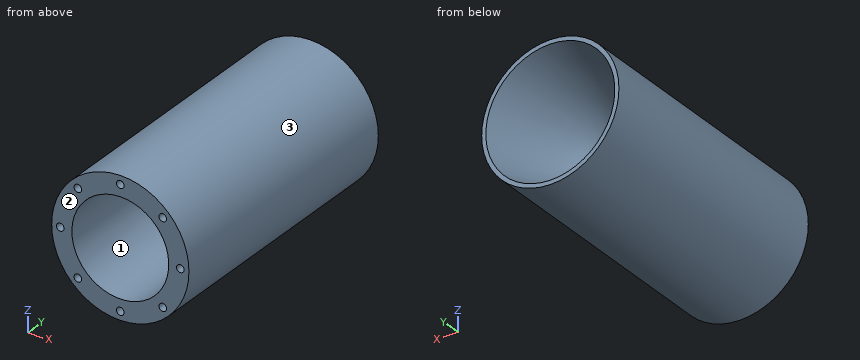
from build123d import *

# Parameters (mm, degrees)
SHORTEN_CHAMBER_75IN_BY = 19.05
CIRPATTERN1_COUNT       = 8


with BuildPart() as part:
    # Sketch1 → Revolve2 (revolve)
    with BuildSketch(Plane.XY, mode=Mode.PRIVATE) as revolve2_sk:
        with BuildLine():
            Line((71.638455479, 109.927347077), (76.2, 109.927347077))
            Line((76.2, 109.927347077), (76.2, -212.127673725))
            Line((76.2, -212.127673725), (53.792460196, -212.127673725))
            Line((53.792460196, -212.127673725), (53.792460196, -59.727673725))
            add(Edge.make_bspline(
                [(53.792460196, -59.727673725), (53.792458964, -59.657143655), (53.791929819, -59.515566601), (53.789553965, -59.181725115), (53.783229362, -58.904955991), (53.77374387, -58.532727986), (53.761100968, -58.21299812), (53.741350135, -57.781754942), (53.711337787, -57.281120398), (53.667125616, -56.688158665), (53.588220936, -55.848640867), (53.488359334, -55.008326363), (53.367608248, -54.172595934), (53.197743271, -53.172585746), (53.002996623, -52.17760333), (52.777307543, -51.188699595), (52.520946634, -50.207649553), (52.240221737, -49.233238259), (51.935281123, -48.266129746), (51.5444702, -47.149295595), (51.050452714, -45.89056894), (50.509666089, -44.651129345), (49.922993248, -43.432862075), (49.291052535, -42.237253796), (48.615057518, -41.066315445), (47.895407794, -39.921133233), (47.134034398, -38.804236825), (46.430801308, -37.85161238), (45.804470174, -37.055832726), (45.263749909, -36.403541893), (44.82605917, -35.894408249), (44.425708405, -35.447153279), (44.092389714, -35.084791811), (43.784856831, -34.760500781), (43.58500461, -34.551710083), (43.355324273, -34.318676923), (43.254715351, -34.217322692), (43.204843203, -34.167450306)],
                knots=[0.082637729, 0.082637729, 0.082637729, 0.082637729, 0.082637729, 0.092574926, 0.102512123, 0.11244932, 0.122386517, 0.132323714, 0.142260911, 0.162135305, 0.182009699, 0.201884093, 0.24163288, 0.261507274, 0.281381668, 0.321130456, 0.360879243, 0.380753637, 0.400628031, 0.440376819, 0.480125606, 0.519874394, 0.559623181, 0.599371969, 0.639120757, 0.678869544, 0.718618332, 0.75836712, 0.798115907, 0.817990301, 0.837864695, 0.857739089, 0.877613483, 0.88755068, 0.897487877, 0.907425074, 0.91736227, 0.91736227, 0.91736227, 0.91736227, 0.91736227], degree=4))
            Line((43.204843203, -34.167450306), (34.597215006, -25.55982211))
            add(Edge.make_bspline(
                [(24.01, 0), (24.010001231, -0.070528647), (24.010530378, -0.21358419), (24.012906064, -0.543182916), (24.019230459, -0.824160397), (24.028715581, -1.194822072), (24.041357875, -1.513435058), (24.0571581, -1.861939603), (24.076113359, -2.193706872), (24.103750974, -2.6180694), (24.143219182, -3.122033947), (24.214231845, -3.879978675), (24.334058818, -4.886450388), (24.510418188, -6.05671076), (24.761817381, -7.385166414), (25.062727465, -8.703574514), (25.412702779, -10.009637208), (25.811293143, -11.301819595), (26.257877555, -12.578099333), (26.75193549, -13.836887482), (27.292605293, -15.076197126), (27.879411561, -16.294609791), (28.511071576, -17.489938791), (29.187464578, -18.661287753), (29.906377287, -19.805743392), (30.668954188, -20.92386007), (31.370099384, -21.874411755), (31.999668317, -22.673445475), (32.535060612, -23.320422132), (32.983187966, -23.84000501), (33.419382225, -24.32981624), (33.846758322, -24.788484383), (34.156490841, -25.113868303), (34.44779216, -25.409649039), (34.547344628, -25.509949925), (34.597215006, -25.55982211)],
                knots=[0.082637729, 0.082637729, 0.082637729, 0.082637729, 0.082637729, 0.092574926, 0.102512123, 0.11244932, 0.122386517, 0.132323714, 0.142260911, 0.152198108, 0.162135305, 0.182009699, 0.201884093, 0.24163288, 0.281381668, 0.321130456, 0.360879243, 0.400628031, 0.440376819, 0.480125606, 0.519874394, 0.559623181, 0.599371969, 0.639120757, 0.678869544, 0.718618332, 0.75836712, 0.798115907, 0.817990301, 0.837864695, 0.857739089, 0.877613483, 0.897487877, 0.907425074, 0.91736227, 0.91736227, 0.91736227, 0.91736227, 0.91736227], degree=4))
            add(Edge.make_bspline(
                [(24.01, 0), (24.010000626, 0.035892652), (24.010538457, 0.11011369), (24.012955849, 0.267641069), (24.019393694, 0.427064117), (24.031465725, 0.646764266), (24.052367213, 0.901433328), (24.086116845, 1.202537273), (24.137431431, 1.542050498), (24.201475827, 1.880996777), (24.278073727, 2.21635442), (24.367255697, 2.549239421), (24.468673539, 2.878092645), (24.582551197, 3.203347041), (24.708128897, 3.523627157), (24.846218103, 3.839666733), (24.995002427, 4.149282184), (25.156944348, 4.454783123), (25.327420631, 4.751301575), (25.513446847, 5.045703861), (25.702720396, 5.325518936), (25.9153376, 5.610727543), (26.0898085, 5.832913647), (26.277277882, 6.049951637), (26.415487374, 6.208641646), (26.581374196, 6.382121779), (26.655452387, 6.458478841), (26.706211329, 6.50923965)],
                knots=[0.082568816, 0.082568816, 0.082568816, 0.082568816, 0.082568816, 0.102426634, 0.122284453, 0.142142271, 0.162000089, 0.201715725, 0.241431362, 0.281146998, 0.320862634, 0.360578271, 0.400293907, 0.440009544, 0.47972518, 0.519440816, 0.559156453, 0.598872089, 0.638587725, 0.678303362, 0.718018998, 0.757734635, 0.797450271, 0.837165907, 0.857023726, 0.876881544, 0.91659718, 0.91659718, 0.91659718, 0.91659718, 0.91659718], degree=4))
            add(Edge.make_bspline(
                [(26.706211329, 6.50923965), (49.172333461, 34.635954224), (71.638455479, 109.927347077)],
                knots=[0, 0, 0, 1, 1, 1], degree=2))
        make_face()
    revolve(revolve2_sk.sketch.rotate(Axis((0, 0, 0), (0, -1, 0)), 90), axis=Axis((0, 0, 0), (0, -1, 0)))

    # shorten_chamber_.75in: a face moved inward by 19.05
    extrude(part.faces().sort_by_distance((60.96, -212.127673725, 0))[0], amount=SHORTEN_CHAMBER_75IN_BY, dir=(0, 1, 0), mode=Mode.SUBTRACT)

    # Sketch4 → 3/8-24 Tapped Hole1 (revolve, cut)
    with BuildSketch(Plane(origin=(66.675, -193.077673725, 0), x_dir=(0, 0, -1), z_dir=(1, 0, 0))):
        Polygon((0, 0), (0, 27.534688714), (4.2164, 25.00122), (4.2164, 0), align=None)
    f_3_8_24_tapped_hole1 = revolve(axis=Axis((66.675, -199.427673725, 0), (0, 1, 0)), mode=Mode.SUBTRACT)

    # CirPattern1: 3/8-24 Tapped Hole1 ×8 about axis
    cirpattern1_axis = Axis((0, 0, 0), (0, 1, 0))
    for i in range(1, CIRPATTERN1_COUNT):
        add(f_3_8_24_tapped_hole1.rotate(cirpattern1_axis, i * 360 / CIRPATTERN1_COUNT), mode=Mode.SUBTRACT)


solid = part.part
For this review, take the finished solid that the model builds, in its own axes (mm). Face numbers are marked on the shaded views. Give positions to 0.01 mm unless a question says otherwise; leave off trailing zeros.
Item 1: Draft analysis for pull direction X (two halves, no side actions). For the marked faces 1, 2 and 3, state which applies: +X half, -X half, draft (parallel to the pull), parting line (faces both ways), or undercut.
Item 2: For line 1 along X through (y, z) = (-181.25, 0); line 2 along X through (y, z) = (-84, 26); line 3 along Z through (x, y) = (23, -58.5), list the stretches that pass through material, from the lowest coordinate up.
Item 3: Insertion check: pin 1 (11 mm diameter, centred on x = -47.15, z = 47.15, fed in from +Y); pin 2 (1.5 mm diameter, centred on x = -33.5, z = -24.5, fed in from +Y); pin 3 (5 mm diameter, centred on y = -9.5, z = -13.5, fed in from -X); pin 4 (5 mm diameter, centred on y = -1, z = 38, fed in from +X). Each pin has a flat end and moves straight along its axis. Give the tip position at first contact, or say it passes through.
Calculated:
1. face 1: undercut
1. face 2: draft
1. face 3: parting line
2. line 1: x = -76.2 to -70.89, -62.46 to -53.79, 53.79 to 62.46, 70.89 to 76.2
2. line 2: x = -71.63 to -47.09, 47.09 to 71.63
2. line 3: z = -72.65 to -48.6, 48.6 to 72.65
3. pin 1: stops at y = 109.93
3. pin 2: stops at y = 31.62
3. pin 3: stops at x = -75.4
3. pin 4: stops at x = 67.43
